Autodesk Inventor part; units mm, degrees
ref_plane "YZ Plane" through (0, 0, 0) normal (1, 0, 0) x (0, 1, 0)
ref_plane "XZ Plane" through (0, 0, 0) normal (0, 1, 0) x (-1, 0, 0)
ref_plane "XY Plane" through (0, 0, 0) normal (0, 0, 1) x (1, 0, 0)
sketch "Skizze1" plane through (0, 0, 0) normal (0, 1, 0) x (-1, 0, 0)
  line L0 (0, 0) -> (1.15, 0) construction
  line L1 (1.15, 0) -> (1.15, -13) construction
  line L2 (1.15, -13) -> (0, -13) construction
  line L3 (0, -13) -> (0, 0) construction
  line L4 (0, -6.5) -> (1.15, -6.5) construction
  line L5 (0.575, -1.85) -> (0.575, -11.15) construction
  line L6 (0.3, -1.7763) -> (1.15, -2.0041) construction
  line L7 (0.85, -2.2343) -> (0, -2.0065) construction
  line L8 (0.3, 0) -> (0.3, -1.7763)
  line L9 (0.3, -11.2237) -> (1.15, -10.9959) construction
  line L10 (0, -10.9935) -> (0.85, -10.7657) construction
  line L11 (0.3, -11.2237) -> (0.3, -13)
  line L12 (0.85, -2.2343) -> (0.85, -10.7657)
  line L13 (0, 0) -> (0.3, 0)
  line L14 (0.3, -1.7763) -> (1.15, -2.0041)
  line L15 (1.15, -10.9959) -> (0.3, -11.2237)
  line L16 (0.3, -13) -> (0, -13)
  line L17 (0, -10.9935) -> (0.85, -10.7657)
  line L18 (0.85, -2.2343) -> (0, -2.0065)
  line L19 (1.15, -2.0041) -> (1.15, -10.9959)
  line L20 (0, -2.0065) -> (0, 0)
  line L21 (0, -10.9935) -> (0, -13)
  point P0 (0.575, -6.5)
  dimension "d0" = 1.15
  dimension "d1" = 13
  dimension "d4" = 9.3
  dimension "d7" = 75
  dimension "d8" = 0.3
  dimension "d9" = 0.3
  dimension "d10" = 75
  dimension "d11" = 0.3
  dimension "d12" = 0.3
extrude "Extrusion1" add sketch "Skizze1" along normal blind 150
equation "\"Biegeradius\" = Stärke"
equation "\"BreiteBiegungsfreistellung\" = Stärke"
equation "\"TiefeBiegungsfreistellung\" = 0.5 * Stärke"
equation "\"GrößeEckenfreistellung\" = 4 * Stärke"
equation "\"MinimalRest\" = 2 * Stärke"
equation "\"Übergangsradius\" = Biegeradius"
equation "\"JacobiRadiusGröße\" = Biegeradius"
equation "\"Abstandsgröße\" = Stärke"
properties part number "Koffer_ankerschiene_15m"
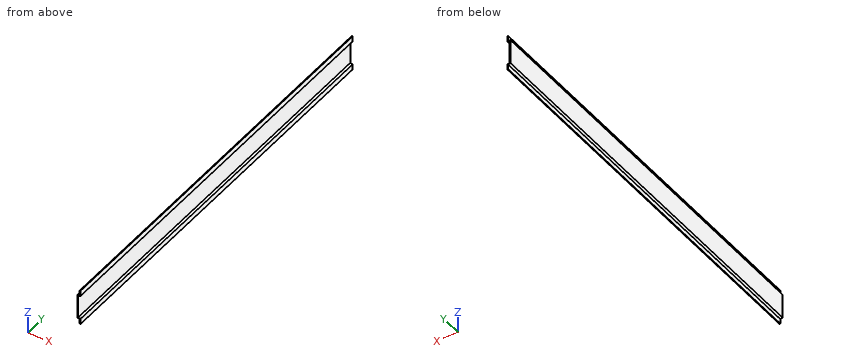
Design review of the part built by this model. Coordinates are the model's own, in mm. Round coordinates to 2 decimals unless told otherwise and drop trailing zeros. Write each loop counter-clockwise with the first axis right and the second up, starting at its lowest first coordinate (ties: lowest second). Pieces come first, ordered by that corner, then holes. Notation, with made-up numbers: (-8.75, 5.25) -> (25.25, 5.25) arc R7 cw to (25.25, 12.25) -> close; hole circle Ø8 at (5, -26). An arc over 180 degrees is marked (long way). One line per question, with ' | ' between items.
(1) Insertion check: P1, Ø1.4, axis at y = 103.5, z = -0.5, coming from the -X side; P2, Ø2.5, axis at y = 72.5, z = -8.5, coming from the +X side. Each pin has a flat end and moves straight along its axis. Give the tip position at first contact, or say it passes through.
Result sheet:
P1: x = -0.3 | P2: x = -0.85
(2) Take a section at C-C, the plane z = -4.5. State the section outline as (x, y) points.
Result sheet:
outline: (-1.15, 0) -> (-0.85, 0) -> (-0.85, 150) -> (-1.15, 150) -> close
(3) Wall thickness on line 1 (Z direction, x = -0.1, y = 68.5); line 2 (X direction, y = 53.5, z = -10.75); line 3 (Z direction, x = -0.5, y = 34): over which ranges is each line inside the solid? List them lowest first. Write a range as [from, to].
Result sheet:
line 1: [-13, -10.97], [-2.03, 0] | line 2: [-1.15, -0.85] | line 3: [-11.17, -10.86], [-2.14, -1.83]
(4) Take a section at B-B, the plane x = -0.65. State the section outline as (y, z) points, and give its area (3 significant figures).
Result sheet:
outline: (0, -11.13) -> (150, -11.13) -> (150, -10.82) -> (0, -10.82) -> close; (0, -2.18) -> (150, -2.18) -> (150, -1.87) -> (0, -1.87) -> close | area: 93.2 mm2
(5) Take a section at A-A, the plane y = 104.5. State the section outline as (x, z) points, and give its area (3 significant figures).
Result sheet:
outline: (-1.15, -11) -> (-0.3, -11.22) -> (-0.3, -13) -> (0, -13) -> (0, -10.99) -> (-0.85, -10.77) -> (-0.85, -2.23) -> (0, -2.01) -> (0, 0) -> (-0.3, 0) -> (-0.3, -1.78) -> (-1.15, -2) -> close | area: 4.29 mm2
